Study the drawing (mm; zero at the part's minimum x, y, z) and answer. A direction names the side the tool comes from. Give positions to 0.01 mm unless a question says otherwise; leave off trailing zeros. Loops run counter-clockwise (first coordinate to the right, second up) from the corner with the lowest first, then second, coordinate; pieces in that order, holes last. Notation, with made-up numbers: M -10.75,-10.5 L 23.25,-10.5 A21 cw 23.25,15.5 Z; hole C -4,-19 d2. An arc over 180 degrees is marked long. Return JSON: item names as keys, results as strings.
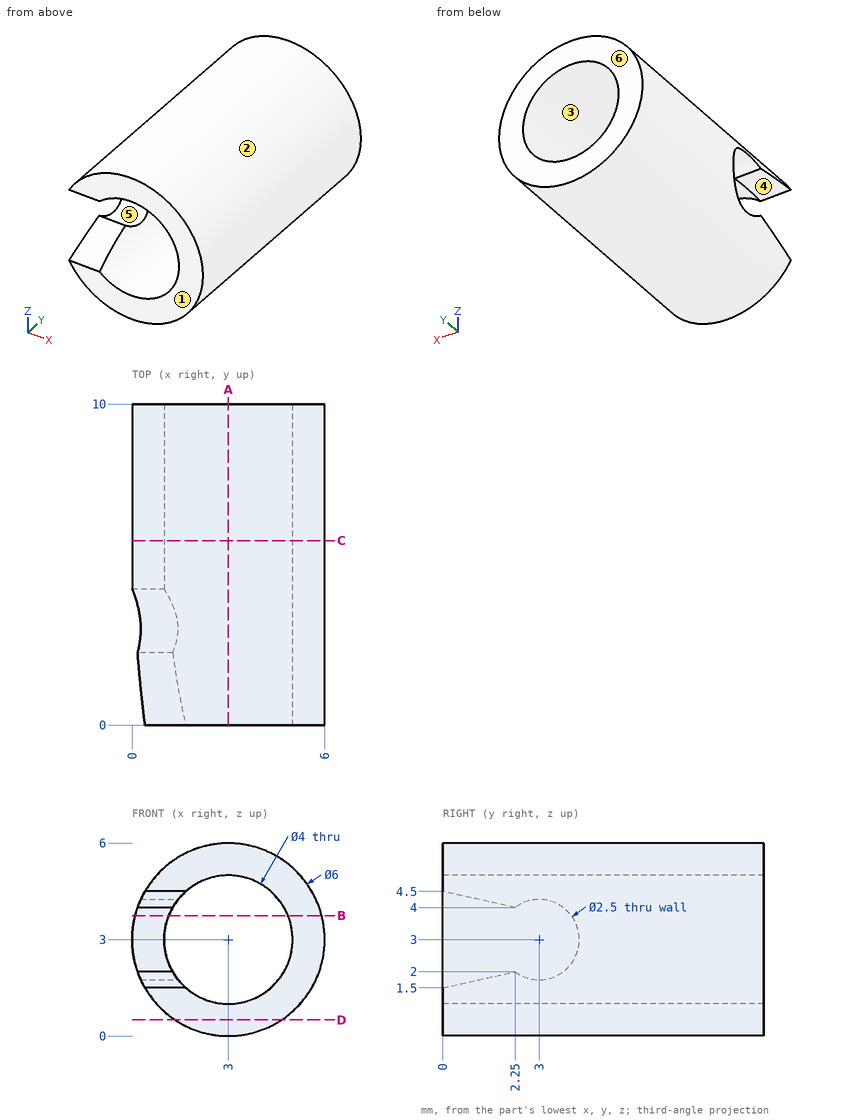
(1) A tool of negligible diameter and unlimited length cuts with its end or side. For the marked faces 4, 5 and 6, from which of +Z, -Z, +X, -X, +Y, -Y can it reach the whole face along a straight path? Write none if from no direction.
Values follow:
{"face 4": "-X, -Y", "face 5": "-X", "face 6": "+Z, -Z, +X, -X, +Y"}
(2) Determine the mould class of the marked faces 1, 2 and 3 for opening direction X: released by +X, released by -X, zero draft, split by the parting line, or undercut.
Values follow:
{"face 1": "zero draft", "face 2": "split by the parting line", "face 3": "undercut"}
(3) The part is cut by section B-B (z = 3.75). Determine the outline of the cut face in (x, y).
Values follow:
{"outline": "M 0.1,4 L 1.15,4 L 1.15,10 L 0.1,10 Z; M 4.85,0 L 5.9,0 L 5.9,10 L 4.85,10 Z"}
(4) The part is cut by section C-C (y = 5.75). Determine the outline of the cut face in (x, z), and give its area (3 significant figures).
Values follow:
{"outline": "C 3,3 d6; hole C 3,3 d4", "area": "15.7 mm²"}
(5) The part is cut by section A-A (x = 3). Determine the outline of the cut face in (y, z).
Values follow:
{"outline": "M 0,0 L 10,0 L 10,1 L 0,1 Z; M 0,5 L 10,5 L 10,6 L 0,6 Z"}
(6) The part is cut by section D-D (z = 0.5). Determine the outline of the cut face in (x, y).
Values follow:
{"outline": "M 1.34,0 L 4.66,0 L 4.66,10 L 1.34,10 Z"}
(7) Given pin 1 (1 mm diameter, centred on y = 4.5, z = 2, fed in from +X); pin 2 (3.5 mm diameter, centred on x = 3, z = 3, fed in from -Y); pin 3 (1 mm diameter, centred on x = 4, y = 5.5, fed in from -Z), each flat-ended and moving along its own axis, determine where each tip first touches the part or whether it passes through.
Values follow:
{"pin 1": "x = 5.96", "pin 2": "through", "pin 3": "z = 0.04"}
(8) Straight lines are drawn through the part: line 1 along Z through (x, y) = (3, 4.5); line 2 along Z through (x, y) = (0.7, 3); line 3 along X through (y, z) = (6, 2). For each, find the intervals that lie inside material, in ascending order.
Values follow:
{"line 1": "0 to 1, 5 to 6", "line 2": "1.07 to 1.75, 4.25 to 4.93", "line 3": "0.17 to 1.27, 4.73 to 5.83"}
